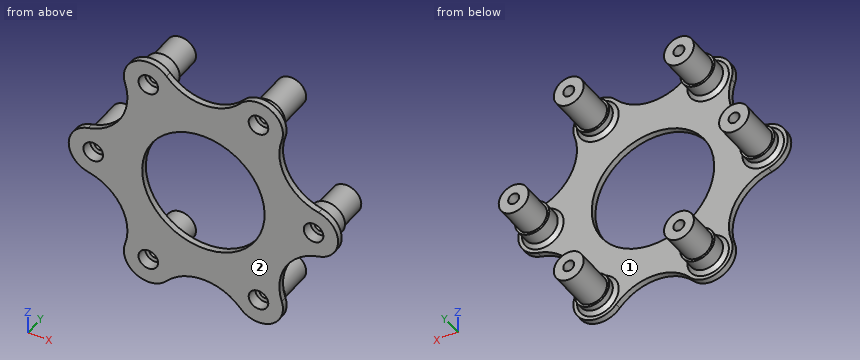
from build123d import *

# Parameters (mm, degrees)
EXTRUDE_1_DEPTH     = 2.5
SKETCH_3_R          = 7
EXTRUDE_2_DEPTH     = 4
CHAMFER_1_SIZE      = 1.5
SKETCH_4_R          = 6.1
EXTRUDE_3_DEPTH     = 16
SKETCH_5_R          = 7
EXTRUDE_4_DEPTH     = 3.3
SKETCH_6_R          = 2.25
CUT_EXTRUDE_1_DEPTH = 78.002745817
SKETCH_7_R          = 4
CUT_EXTRUDE_2_DEPTH = 4.5
SKETCH_8_R          = 25
CUT_EXTRUDE_3_DEPTH = 10


with BuildPart() as part:
    # 草图2 → 凸台-拉伸1 (new body)
    with BuildSketch(Plane(origin=(0, 0, 0), x_dir=(1, 0, 0), z_dir=(0, 1, 0))):
        with BuildLine():
            ThreePointArc((-47.091925455, 9.778744699), (-55, -1.253e-06), (-47.091923006, -9.778745223))
            ThreePointArc((-47.091923006, -9.778745223), (-33.750000065, -19.485571473), (-32.014603203, -35.893428778))
            ThreePointArc((-32.014603203, -35.893428778), (-27.500000081, -47.631397162), (-15.077319674, -45.672174193))
            ThreePointArc((-15.077319674, -45.672174193), (-9.8e-08, -38.97114317), (15.077319542, -45.672174048))
            ThreePointArc((15.077319542, -45.672174048), (27.500000118, -47.63139714), (32.014603117, -35.893428511))
            ThreePointArc((32.014603117, -35.893428511), (33.750000078, -19.485571451), (47.091922781, -9.778745271))
            ThreePointArc((47.091922781, -9.778745271), (55, -2.05e-07), (47.091923183, 9.778745185))
            ThreePointArc((47.091923183, 9.778745185), (33.750000105, 19.485571404), (32.01460321, 35.893428798))
            ThreePointArc((32.01460321, 35.893428798), (27.499999984, 47.631397217), (15.077319539, 45.672174044))
            ThreePointArc((15.077319539, 45.672174044), (1.8e-08, 38.97114317), (-15.077319515, 45.672174018))
            ThreePointArc((-15.077319515, 45.672174018), (-27.5000001, 47.63139715), (-32.014603117, 35.893428511))
            ThreePointArc((-32.014603117, 35.893428511), (-33.750000761, 19.485570266), (-47.091925455, 9.778744699))
        make_face()
    extrude(amount=EXTRUDE_1_DEPTH)

    # 草图3 → 凸台-拉伸2 (add)
    with BuildSketch(Plane(origin=(0, 2.5, 0), x_dir=(1, 0, 0), z_dir=(0, 1, 0))):
        with Locations(Location((-22.5, 38.97114317, 0), (0, 0, 270))):
            Circle(SKETCH_3_R)
        with Locations(Location((22.5, 38.97114317, 0), (0, 0, 270))):
            Circle(SKETCH_3_R)
        with Locations(Location((45, 0, 0), (0, 0, 270))):
            Circle(SKETCH_3_R)
        with Locations(Location((22.5, -38.97114317, 0), (0, 0, 270))):
            Circle(SKETCH_3_R)
        with Locations(Location((-22.5, -38.97114317, 0), (0, 0, 270))):
            Circle(SKETCH_3_R)
        with Locations(Location((-45, 0, 0), (0, 0, 270))):
            Circle(SKETCH_3_R)
    extrude(amount=EXTRUDE_2_DEPTH)

    # 倒角1
    chamfer_1_edges = [part.edges().sort_by_distance(p)[0] for p in [
        (-22.5, 2.5, -45.97114317),
        (22.5, 2.5, -45.97114317),
        (45, 2.5, -7),
        (22.5, 2.5, 31.97114317),
        (-22.5, 2.5, 31.97114317),
        (-45, 2.5, -7),
    ]]
    chamfer(chamfer_1_edges, length=CHAMFER_1_SIZE)

    # 草图4 → 凸台-拉伸3 (add)
    with BuildSketch(Plane(origin=(0, 6.5, 0), x_dir=(1, 0, 0), z_dir=(0, 1, 0))):
        with Locations(Location((-22.5, 38.97114317, 0), (0, 0, 270))):
            Circle(SKETCH_4_R)
        with Locations(Location((22.5, 38.97114317, 0), (0, 0, 270))):
            Circle(SKETCH_4_R)
        with Locations(Location((45, 0, 0), (0, 0, 270))):
            Circle(SKETCH_4_R)
        with Locations(Location((22.5, -38.97114317, 0), (0, 0, 270))):
            Circle(SKETCH_4_R)
        with Locations(Location((-22.5, -38.97114317, 0), (0, 0, 270))):
            Circle(SKETCH_4_R)
        with Locations(Location((-45, 0, 0), (0, 0, 270))):
            Circle(SKETCH_4_R)
    extrude(amount=EXTRUDE_3_DEPTH)

    # 草图5 → 凸台-拉伸4 (add)
    with BuildSketch(Plane(origin=(0, 6.5, 0), x_dir=(1, 0, 0), z_dir=(0, 1, 0))):
        with Locations(Location((-22.5, 38.97114317, 0), (0, 0, 270))):
            Circle(SKETCH_5_R)
        with Locations(Location((45, 0, 0), (0, 0, 270))):
            Circle(SKETCH_5_R)
        with Locations(Location((-22.5, -38.97114317, 0), (0, 0, 270))):
            Circle(SKETCH_5_R)
    extrude(amount=EXTRUDE_4_DEPTH)

    # 草图6 → 切除-拉伸1 (cut, through all)
    with BuildSketch(Plane.XZ):
        with Locations(Location((-22.5, 38.97114317, 0), (0, 0, 270))):
            Circle(SKETCH_6_R)
        with Locations(Location((22.5, 38.97114317, 0), (0, 0, 270))):
            Circle(SKETCH_6_R)
        with Locations(Location((45, 0, 0), (0, 0, 270))):
            Circle(SKETCH_6_R)
        with Locations(Location((22.5, -38.97114317, 0), (0, 0, 270))):
            Circle(SKETCH_6_R)
        with Locations(Location((-22.5, -38.97114317, 0), (0, 0, 270))):
            Circle(SKETCH_6_R)
        with Locations(Location((-45, 0, 0), (0, 0, 270))):
            Circle(SKETCH_6_R)
    extrude(amount=-CUT_EXTRUDE_1_DEPTH, mode=Mode.SUBTRACT)

    # 草图7 → 切除-拉伸2 (cut)
    with BuildSketch(Plane.XZ):
        with Locations(Location((-22.5, 38.97114317, 0), (0, 0, 270))):
            Circle(SKETCH_7_R)
        with Locations(Location((22.5, 38.97114317, 0), (0, 0, 270))):
            Circle(SKETCH_7_R)
        with Locations(Location((45, 0, 0), (0, 0, 270))):
            Circle(SKETCH_7_R)
        with Locations(Location((22.5, -38.97114317, 0), (0, 0, 270))):
            Circle(SKETCH_7_R)
        with Locations(Location((-22.5, -38.97114317, 0), (0, 0, 270))):
            Circle(SKETCH_7_R)
        with Locations(Location((-45, 0, 0), (0, 0, 270))):
            Circle(SKETCH_7_R)
    extrude(amount=-CUT_EXTRUDE_2_DEPTH, mode=Mode.SUBTRACT)

    # 草图8 → 切除-拉伸3 (cut)
    with BuildSketch(Plane(origin=(0, 2.5, 0), x_dir=(1, 0, 0), z_dir=(0, 1, 0))):
        with Locations(Location((0, 0, 0), (0, 0, 270))):
            Circle(SKETCH_8_R)
    extrude(amount=-CUT_EXTRUDE_3_DEPTH, mode=Mode.SUBTRACT)


solid = part.part
Geometry: final body of the model. Coordinates: model frame, mm. Face numbers are marked on the shaded views. Give positions to 0.01 mm unless a question says otherwise; leave off trailing zeros. Write each loop counter-clockwise with the first axis right and the second up, starting at its lowest first coordinate (ties: lowest second). Pieces come first, ordered by that corner, then holes. Notation, with made-up numbers: (18, 45.5) -> (22, 45.5) arc R28 ccw to (22, 69.5) -> close; hole circle Ø6 at (-27, -9.5). An arc over 180 degrees is marked (long way). Answer as a JSON object with one key per item and string values.
1. Contact query for flat-ended pins moving along their axis: pin 1 (2.5 mm diameter, centred on x = 45, z = 0, fed in from +Y); pin 2 (1.5 mm diameter, centred on x = 16.5, y = 12, fed in from +Z); pin 3 (2.5 mm diameter, centred on x = -22, z = 40, fed in from -Y); pin 4 (1.5 mm diameter, centred on x = -28, z = 19.5, fed in from +Y). Output: stop coordinate, or through.
Ans:
{"pin 1": "passes through", "pin 2": "stops at z = 42.08", "pin 3": "stops at y = 4.5", "pin 4": "stops at y = 2.5"}
2. Cut plane A-A on y = 20.5. Count the separate pieces of the cut face and the enclosed holes in it, and give its area (3 significant figures).
Ans:
{"separate pieces": "6", "enclosed holes": "6", "area": "606 mm^2"}
3. Cut plane B-B on x = 0. Output: boundary loops of the cut face in (y, z), and give its area (3 significant figures).
Ans:
{"outline": "(0, -38.97) -> (2.5, -38.97) -> (2.5, -25) -> (0, -25) -> close; (0, 25) -> (2.5, 25) -> (2.5, 38.97) -> (0, 38.97) -> close", "area": "69.9 mm^2"}
4. Mould query, pull axis X, two halves, no side actions, for the marked faces 1 and 2. Classes: pulls with the +X half, pulls with the -X half, needs draft (parallel to the pull), parting line crosses it, or undercut.
Ans:
{"face 1": "undercut", "face 2": "needs draft"}
5. Cut plane D-D on x = 45. Output: boundary loops of the cut face in (y, z), and give its area (3 significant figures).
Ans:
{"outline": "(0, -10.34) -> (2.5, -10.34) -> (2.5, -8.5) -> (4, -7) -> (9.8, -7) -> (9.8, -6.1) -> (22.5, -6.1) -> (22.5, -2.25) -> (4.5, -2.25) -> (4.5, -4) -> (0, -4) -> close; (0, 4) -> (4.5, 4) -> (4.5, 2.25) -> (22.5, 2.25) -> (22.5, 6.1) -> (9.8, 6.1) -> (9.8, 7) -> (4, 7) -> (2.5, 8.5) -> (2.5, 10.34) -> (0, 10.34) -> close", "area": "194 mm^2"}
6. Cut plane C-C on z = 11. Output: boundary loops of the cut face in (x, y), and give its area (3 significant figures).
Ans:
{"outline": "(-43.27, 0) -> (-22.45, 0) -> (-22.45, 2.5) -> (-43.27, 2.5) -> close; (22.45, 0) -> (43.27, 0) -> (43.27, 2.5) -> (22.45, 2.5) -> close", "area": "104 mm^2"}
7. Ray query, probe 1 along X at (y, z) = (16, 0); probe 2 along Z at (x, y) = (21, 19.75); probe 3 along X at (y, z) = (6.25, 38.5). Return the intervals inside material, ascending. Write a range as from..to.
Ans:
{"probe 1": "x = -51.1..-47.25, -42.75..-38.9, 38.9..42.75, 47.25..51.1", "probe 2": "z = -44.88..-40.65, -37.29..-33.06, 33.06..37.29, 40.65..44.88", "probe 3": "x = -29.48..-24.7, -20.3..-15.52, 15.52..20.3, 24.7..29.48"}
